The listing builds one solid part. Answer for the finished solid, in the listing's coordinates (mm). A direction names the side the tool comes from. Give positions to 0.01 mm unless a question says otherwise; leave off trailing zeros. Order: outer loops, then holes, each group sorted by start corner. A loop starts at its lowest first (then second) coordinate and runs counter-clockwise, first axis right, second up. Notation, with made-up numbers: (60, 66) - (117, 66) arc R9 cw to (117, 76) - close; hole circle Ø3 at (44.25, 25.25). An arc over 180 degrees is marked (long way). Answer in a Markdown table with one row per item.
from build123d import *

# Parameters (mm, degrees)
SKETCH1_W               = 120
SKETCH1_H               = 80
BOSS_EXTRUDE1_DEPTH     = 15
SKETCH2_R               = 25
BOSS_EXTRUDE2_DEPTH     = 35
SKETCH3_R               = 15
CUT_EXTRUDE1_DEPTH      = 88.749643874
SKETCH4_R               = 4
CUT_EXTRUDE2_DEPTH      = 81.156097709
LPATTERN1_COUNT         = 2
LPATTERN1_PITCH         = 100
MIRROR1_COPY_1_SKETCH_R = 4
MIRROR1_COPY_1_DEPTH    = 81.156097709
SKETCH5_R               = 2.5
CUT_EXTRUDE3_DEPTH      = 12
CIRPATTERN1_COUNT       = 4
CHAMFER1_SIZE           = 1.5
CHAMFER2_SIZE           = 1
RIB6_REACH              = 89.75
SKETCH8_2_WALL_W        = 204.614781474
SKETCH8_2_WALL_H        = 8
RIB7_REACH              = 89.75
SKETCH9_WALL_W          = 204.614781474
SKETCH9_WALL_H          = 8
FILLET2_R               = 2


with BuildPart() as part:
    # Sketch1 → Boss-Extrude1 (new body)
    with BuildSketch(Plane.XY):
        Rectangle(SKETCH1_W, SKETCH1_H)
    extrude(amount=BOSS_EXTRUDE1_DEPTH)

    # Sketch2 → Boss-Extrude2 (add)
    with BuildSketch(Plane.XY.offset(15)):
        Circle(SKETCH2_R)
    extrude(amount=BOSS_EXTRUDE2_DEPTH)

    # Sketch3 → Cut-Extrude1 (cut, through all)
    with BuildSketch(Plane.XY.offset(50)):
        Circle(SKETCH3_R)
    extrude(amount=-CUT_EXTRUDE1_DEPTH, mode=Mode.SUBTRACT)

    # Sketch4 → Cut-Extrude2 (cut, through all)
    with BuildSketch(Plane.XY.offset(15)):
        with Locations((-50, 30)):
            Circle(SKETCH4_R)
    cut_extrude2 = extrude(amount=-CUT_EXTRUDE2_DEPTH, mode=Mode.SUBTRACT)

    # LPattern1: Cut-Extrude2 ×2
    with Locations(*[(i * LPATTERN1_PITCH, 0, 0) for i in range(1, LPATTERN1_COUNT)]):
        add(cut_extrude2, mode=Mode.SUBTRACT)

    # Mirror1: Cut-Extrude2 across plane
    add(cut_extrude2.mirror(Plane.ZX), mode=Mode.SUBTRACT)

    # Mirror1 copy 1 sketch → Mirror1 copy 1 (cut, through all)
    with BuildSketch(Plane(origin=(100, 0, 15), x_dir=(1, 0, 0), z_dir=(0, 0, 1))):
        with Locations((-50, -30)):
            Circle(MIRROR1_COPY_1_SKETCH_R)
    extrude(amount=-MIRROR1_COPY_1_DEPTH, mode=Mode.SUBTRACT)

    # Sketch5 → Cut-Extrude3 (cut)
    with BuildSketch(Plane.XY.offset(50)):
        with Locations((20, 0)):
            Circle(SKETCH5_R)
    cut_extrude3 = extrude(amount=-CUT_EXTRUDE3_DEPTH, mode=Mode.SUBTRACT)

    # CirPattern1: Cut-Extrude3 ×4 about axis
    cirpattern1_axis = Axis((0, 0, 0), (0, 0, 1))
    for i in range(1, CIRPATTERN1_COUNT):
        add(cut_extrude3.rotate(cirpattern1_axis, i * 360 / CIRPATTERN1_COUNT), mode=Mode.SUBTRACT)

    # Chamfer1
    chamfer1_edges = [part.edges().sort_by_distance(p)[0] for p in [
        (-25, 0, 50),
    ]]
    chamfer(chamfer1_edges, length=CHAMFER1_SIZE)

    # Chamfer2
    chamfer2_edges = [part.edges().sort_by_distance(p)[0] for p in [
        (-15, 0, 50),
    ]]
    chamfer(chamfer2_edges, length=CHAMFER2_SIZE)

    # Sketch8_2 wall → Rib6 (add, up to next)
    with BuildSketch(Plane(origin=(0, 30.75, 27.5), x_dir=(0, -0.387232484355, 0.921982105607), z_dir=(0, -0.921982105607, -0.387232484355)), mode=Mode.PRIVATE) as rib6_sk1:
        Rectangle(SKETCH8_2_WALL_W, SKETCH8_2_WALL_H)
    rib6_tool1 = extrude(rib6_sk1.sketch, amount=RIB6_REACH, mode=Mode.PRIVATE) - part.part
    add(rib6_tool1.solids().sort_by_distance((0, 30.75, 27.5))[0])

    # Sketch9 wall → Rib7 (add, up to next)
    with BuildSketch(Plane(origin=(0, -30.75, 27.5), x_dir=(0, 0.387232484355, 0.921982105607), z_dir=(0, -0.921982105607, 0.387232484355)), mode=Mode.PRIVATE) as rib7_sk1:
        Rectangle(SKETCH9_WALL_W, SKETCH9_WALL_H)
    rib7_tool1 = extrude(rib7_sk1.sketch, amount=-RIB7_REACH, mode=Mode.PRIVATE) - part.part
    add(rib7_tool1.solids().sort_by_distance((0, -30.75, 27.5))[0])

    # Fillet2
    fillet2_edges = [part.edges().sort_by_distance(p)[0] for p in [
        (60, 0, 0),
    ]]
    fillet(fillet2_edges, radius=FILLET2_R)


solid = part.part
Item 1: Determine the mould class of faces 4 (the face through (-5.42, -24.406, 31.516)), 5 (the face through (0, -20, 38)), 6 (the face through (-28, 1, 15)), 7 (the face through (-0.1, 17.5, 44.1)) for opening direction X: pulls with the +X half, pulls with the -X half, needs draft (parallel to the pull), parting line crosses it, or undercut.
Answer block:
| item | result |
|---|---|
| face 4 | parting line crosses it |
| face 5 | undercut |
| face 6 | needs draft |
| face 7 | undercut |
Item 2: Find section D-D on z = 13.5. Write down the section's boundary in (x, y).
Answer block:
| item | result |
|---|---|
| outline | (-60, -40) - (60, -40) - (60, 40) - (-60, 40) - close; hole circle Ø8 at (-50, -30); hole circle Ø8 at (-50, 30); hole circle Ø30 at (0, 0); hole circle Ø8 at (50, -30); hole circle Ø8 at (50, 30) |
Item 3: Find section A-A on x = -50. Write down the section's boundary in (y, z), then the cut area to 3 significant figures.
Answer block:
| item | result |
|---|---|
| outline | (-40, 0) - (-34, 0) - (-34, 15) - (-40, 15) - close; (-26, 0) - (26, 0) - (26, 15) - (-26, 15) - close; (34, 0) - (40, 0) - (40, 15) - (34, 15) - close |
| area | 960 mm² |
Item 4: Find section B-B on z = 28.5. Write down the section's boundary in (x, y).
Answer block:
| item | result |
|---|---|
| outline | (-4, -30.33) - (4, -30.33) - (4, -24.68) arc R25 ccw to (4, 24.68) - (4, 30.33) - (-4, 30.33) - (-4, 24.68) arc R25 ccw to (-4, -24.68) - close; hole circle Ø30 at (0, 0) |
Item 5: Consider line 1 (Y direction, x = -50, z = 10.25); line 2 (X direction, y = -20, z = 41.5); line 3 (Y direction, x = 47.5, z = 10). Determine where each line is inside the solid, lowest interval first.
Answer block:
| item | result |
|---|---|
| line 1 | -40 to -34, -26 to 26, 34 to 40 |
| line 2 | -15 to -2.5, 2.5 to 15 |
| line 3 | -40 to -33.12, -26.88 to 26.88, 33.12 to 40 |
Item 6: Each of these flat-tipped pins is pushed along its axis until it touches: P1, Ø6, axis at x = -38, y = -1, coming from the -Z side; P2, Ø2.5, axis at x = -1, y = 20, coming from the +Z side; P3, Ø13, axis at x = -50, y = 30, coming from the +Z side; P4, Ø9, axis at y = 32.5, z = 22.5, coming from the -X side. Where does it stop, or does it pass through?
Answer block:
| item | result |
|---|---|
| P1 | z = 0 |
| P2 | z = 38 |
| P3 | z = 15 |
| P4 | x = -4 |
Item 7: Find section C-C on y = 0. Write down the section's boundary in (x, z).
Answer block:
| item | result |
|---|---|
| outline | (-60, 0) - (-15, 0) - (-15, 49) - (-16, 50) - (-17.5, 50) - (-17.5, 38) - (-22.5, 38) - (-22.5, 50) - (-23.5, 50) - (-25, 48.5) - (-25, 15) - (-60, 15) - close; (15, 0) - (58, 0) arc R2 ccw to (60, 2) - (60, 15) - (25, 15) - (25, 48.5) - (23.5, 50) - (22.5, 50) - (22.5, 38) - (17.5, 38) - (17.5, 50) - (16, 50) - (15, 49) - close |
Item 8: Which of the six approach directions +Z, -Z, +X, -X, +Y, -Y give full straight-line access (tool end or side, diameter ignored) to faces 1 (the face through (-1, 40, 7)), 2 (the face through (4, 28, 24)), 3 (the face through (-20, 0, 38))?
Answer block:
| item | result |
|---|---|
| face 1 | +Z, -Z, +X, -X, +Y |
| face 2 | +Z, +X, +Y |
| face 3 | +Z |
